Model file for the job. Use its own axes, mm. Coordinates: 2 decimals unless noted, no trailing zeros. Loops run counter-clockwise (first coordinate to the right, second up) from the corner with the lowest first, then second, coordinate; pieces in that order, holes last. Notation, with made-up numbers: (5.5, -21.5) - (37.5, -21.5) arc R10 cw to (37.5, -13.5) - close; hole circle Ø10 at (-16.75, 12.25). An arc over 180 degrees is marked (long way). Write each question's results on one line, items separated by ' | '. Start each with the question number.
```python
from build123d import *

# Parameters (mm, degrees)
SKETCH1_R           = 9.398
BOSS_EXTRUDE1_DEPTH = 74.93
SKETCH2_R           = 6.223
CUT_EXTRUDE1_DEPTH  = 69.088
BOSS_EXTRUDE2_START = -74.93
BOSS_EXTRUDE2_DEPTH = 74.93
CUT_EXTRUDE6_DEPTH  = 4.318
CIRPATTERN2_COUNT   = 6


with BuildPart() as part:
    # Sketch1 → Boss-Extrude1 (new body)
    with BuildSketch(Plane(origin=(0, 0, 0), x_dir=(1, 0, 0), z_dir=(0, 1, 0))):
        with Locations(Location((0, 0, 0), (0, 0, 270))):
            Circle(SKETCH1_R)
    extrude(amount=BOSS_EXTRUDE1_DEPTH)

    # Sketch2 → Cut-Extrude1 (cut)
    with BuildSketch(Plane(origin=(0, 74.93, 0), x_dir=(1, 0, 0), z_dir=(0, 1, 0))):
        with Locations(Location((0, 0, 0), (0, 0, 270))):
            Circle(SKETCH2_R)
    extrude(amount=-CUT_EXTRUDE1_DEPTH, mode=Mode.SUBTRACT)

    # Sketch7 → Boss-Extrude2 (add)
    with BuildSketch(Plane(origin=(0, 74.93, 0), x_dir=(1, 0, 0), z_dir=(0, 1, 0)).offset(BOSS_EXTRUDE2_START)):
        with BuildLine():
            ThreePointArc((-8.138906715, 4.699000052), (-4.698999978, 8.138906757), (-9e-09, 9.398))
            Line((-9e-09, 9.398), (-5.42593783, 9.398))
            Line((-5.42593783, 9.398), (-8.138906715, 4.699000052))
        make_face()
        with BuildLine():
            ThreePointArc((-9e-09, 9.398), (4.69899997, 8.138906762), (8.138906715, 4.699000052))
            Line((8.138906715, 4.699000052), (5.42593783, 9.398))
            Line((5.42593783, 9.398), (-9e-09, 9.398))
        make_face()
        with BuildLine():
            Line((8.138906731, -4.699000024), (10.85187566, 0))
            Line((10.85187566, 0), (8.138906715, 4.699000052))
            ThreePointArc((8.138906715, 4.699000052), (9.077770908, 2.432381415), (9.398, 0))
            ThreePointArc((9.398, 0), (9.077770912, -2.432381399), (8.138906731, -4.699000024))
        make_face()
        with BuildLine():
            Line((5.42593783, -9.398), (8.138906731, -4.699000024))
            ThreePointArc((8.138906731, -4.699000024), (4.698999988, -8.138906752), (0, -9.398))
            Line((0, -9.398), (5.42593783, -9.398))
        make_face()
        with BuildLine():
            Line((-5.42593783, -9.398), (0, -9.398))
            ThreePointArc((0, -9.398), (-4.699000032, -8.138906726), (-8.138906781, -4.698999937))
            Line((-8.138906781, -4.698999937), (-5.42593783, -9.398))
        make_face()
        with BuildLine():
            ThreePointArc((-8.138906781, -4.698999937), (-9.398, 6.6e-08), (-8.138906715, 4.699000052))
            Line((-8.138906715, 4.699000052), (-10.85187566, 0))
            Line((-10.85187566, 0), (-8.138906781, -4.698999937))
        make_face()
    extrude(amount=BOSS_EXTRUDE2_DEPTH)

    # Sketch8 → Cut-Extrude6 (cut)
    with BuildSketch(Plane.XZ):
        Polygon((-1.75976362, -5.588), (-2.492998462, -4.318), (-3.959468146, -4.318), (-4.692702988, -5.588), (-3.959468146, -6.858), (-2.492998462, -6.858), align=None)
    cut_extrude6 = extrude(amount=-CUT_EXTRUDE6_DEPTH, mode=Mode.SUBTRACT)

    # CirPattern2: Cut-Extrude6 ×6 about axis
    cirpattern2_axis = Axis((0.06001178, 0, 0.103943452), (0, 1, 0))
    for i in range(1, CIRPATTERN2_COUNT):
        add(cut_extrude6.rotate(cirpattern2_axis, i * 360 / CIRPATTERN2_COUNT), mode=Mode.SUBTRACT)


solid = part.part
```
Q1. Pin check, flat tips, straight feed: pin 1 (1.5 mm diameter, centred on y = 16, z = 2, fed in from -X); pin 2 (1.5 mm diameter, centred on x = 2, z = 1.5, fed in from +Y); pin 3 (0.8 mm diameter, centred on x = 3, z = -6, fed in from -Y). Stop position of each tip, or through.
Q2. Cut at A-A (y = 60.5). List the corners of the cut face in (x, z).
Q3. Cut at C-C (z = -3.5). List the corners of the cut face in (x, y), and give its area (3 significant figures).
Q4. Cut at D-D (z = 7.75). List the corners of the cut face in (x, y), and give its area (3 significant figures).
Q5. Mould opens along X. For faces 1 (the flat face through (0, 5.842, 0)), 2 (the flat face through (0, 37, -9.398)) say: +X half, -X half, draft (parallel to the pull), parting line (faces both ways), or undercut.
Q6. Drill centre lines: L1, parallel to X at y = 55.5, z = 0; L2, parallel to Y at x = 1.25, z = -3.5; L3, parallel to X at y = 21, z = 0.25. Where is each one in solid material? Low to high. Write a range as from..to.
Q7. Cut at B-B (x = 0). List the corners of the cut face in (y, z).
Check result:
1) pin 1: x = -10.13 | pin 2: y = 5.84 | pin 3: y = 4.32
2) outline: (-10.85, 0) - (-5.43, -9.4) - (5.43, -9.4) - (10.85, 0) - (5.43, 9.4) - (-5.43, 9.4) - close; hole circle Ø12.45 at (0, 0)
3) outline: (-8.83, 0) - (8.83, 0) - (8.83, 74.93) - (5.15, 74.93) - (5.15, 5.84) - (-5.15, 5.84) - (-5.15, 74.93) - (-8.83, 74.93) - close | area: 612 mm²
4) outline: (-6.38, 0) - (6.38, 0) - (6.38, 74.93) - (-6.38, 74.93) - close | area: 956 mm²
5) face 1: undercut | face 2: draft
6) L1: -10.85..-6.22, 6.22..10.85 | L2: 0..5.84 | L3: -10.71..-6.22, 6.22..10.71
7) outline: (0, -9.4) - (74.93, -9.4) - (74.93, -6.22) - (5.84, -6.22) - (5.84, 6.22) - (74.93, 6.22) - (74.93, 9.4) - (0, 9.4) - close
